Autodesk Inventor part; units mm, degrees
ref_plane "Work Plane2" through (-40.9959, 0.8639, 22.2359) normal (0, 0, 1) x (1, 0, 0)
ref_plane "YZ Plane" through (0, 0, 0) normal (1, 0, 0) x (0, 1, 0)
ref_plane "XZ Plane" through (0, 0, 0) normal (0, 1, 0) x (-1, 0, 0)
ref_plane "Work Plane1" through (0, 0, 10) normal (0, 0, 1) x (1, 0, 0)
sketch "Sketch1" plane through (0, 0, 10) normal (0, 0, 1) x (1, 0, 0)
  line L0 (-4.0299, -0.3538) -> (-2.2322, 1.4439) construction
  arc A0 (-1.4439, 2.2322) -> (-2.2322, 1.4439) centre (-0.9299, 0.9299) ccw construction
  line L1 (-1.4439, 2.2322) -> (0.3538, 4.0299) construction
  line L2 (-37.8299, 42.8299) -> (-37.8299, 37.8299) construction
  line L3 (-37.8299, 37.8299) -> (-42.9208, 37.8299) construction
  line L4 (-37.8299, 42.2137) -> (-37.8299, 45.8299) construction
  line L5 (-37.8299, 45.8299) -> (-4.0299, 45.8299) construction
  line L6 (-4.0299, 45.8299) -> (-4.0299, 42.2137) construction
  line L7 (-4.0299, 4.0299) -> (0.3538, 4.0299)
  circle A1 centre (-20.9299, 20.9299) radius 17.5
  line L8 (-20.9299, 58.9723) -> (17.1124, 20.9299) construction
  line L9 (17.1124, 20.9299) -> (-20.9299, -17.1124) construction
  line L10 (-20.9299, -17.1124) -> (-58.9723, 20.9299) construction
  line L11 (-58.9723, 20.9299) -> (-20.9299, 58.9723) construction
  line L12 (-20.9299, 58.9723) -> (-20.9299, -17.1124) construction
  line L13 (17.1124, 20.9299) -> (-58.9723, 20.9299) construction
  line L14 (-20.9299, 58.9723) -> (32.8701, 58.9723) construction
  line L15 (-43.4299, 43.4299) -> (1.5701, 43.4299) construction
  line L16 (1.5701, 43.4299) -> (1.5701, -1.5701) construction
  line L17 (1.5701, -1.5701) -> (-43.4299, -1.5701) construction
  line L18 (-43.4299, -1.5701) -> (-43.4299, 43.4299) construction
  line L19 (-43.4299, 43.4299) -> (1.5701, -1.5701) construction
  line L20 (1.5701, 43.4299) -> (-43.4299, -1.5701) construction
  line L21 (-43.4299, 5.3876) -> (-43.4299, 36.4723)
  line L22 (-43.4299, 36.4723) -> (-36.4723, 43.4299)
  line L23 (-36.4723, 43.4299) -> (-5.3876, 43.4299)
  line L24 (-5.3876, 43.4299) -> (1.5701, 36.4723)
  line L25 (1.5701, 36.4723) -> (1.5701, 5.3876)
  line L26 (1.5701, 5.3876) -> (-5.3876, -1.5701)
  line L27 (-5.3876, -1.5701) -> (-36.4723, -1.5701)
  line L28 (-36.4723, -1.5701) -> (-43.4299, 5.3876)
  line L29 (-4.0299, 42.2137) -> (-37.8299, 42.2137)
  line L30 (-4.0299, -0.3538) -> (-4.0299, 4.0299)
  point P0 (-37.8299, 4.0299)
  point P1 (-20.9299, 20.9299)
  dimension "d18" = 53.8
  dimension "d19" = 45
  dimension "d20" = 53.8
  dimension "d21" = 45
  dimension "d22" = 45
extrude "Extrusion1" add sketch "Sketch1" along normal blind 8
sketch "Sketch2" plane through (0, 0, 18) normal (0, 0, 1) x (1, 0, 0)
  circle A0 centre (-35.9299, 35.9299) radius 3.0099 construction
  circle A1 centre (-5.93, 35.9299) radius 3.0099 construction
  circle A2 centre (-5.93, 5.93) radius 3.0099 construction
  circle A3 centre (-35.9299, 5.93) radius 3.0099 construction
  circle A4 centre (-35.9299, 35.9299) radius 2.95
  circle A5 centre (-5.93, 35.9299) radius 2.95
  circle A6 centre (-5.93, 5.93) radius 2.95
  circle A7 centre (-35.9299, 5.93) radius 2.95
  point P0 (0, 0)
  dimension "d1" = 5.9
  dimension "d31" = 5.9
  dimension "d32" = 5.9
  dimension "d33" = 5.9
ref_plane "Work Plane2" through (-40.9959, 0.8639, 22.2359) normal (0, 0, 1) x (1, 0, 0)
extrude "Extrusion2" add sketch "Sketch2" along normal blind 8
sketch "Sketch3" plane through (0, 0, 10) normal (0, 0, -1) x (-1, 0, 0)
  line L0 (37.8299, -0.4701) -> (37.8299, 4.0299) construction
  line L1 (4.0299, 4.0299) -> (4.0299, -0.4701) construction
  line L2 (37.8299, -0.4701) -> (37.8299, 1.1886) construction
  line L3 (4.0299, -3.9701) -> (4.0299, -0.3538) construction
  line L4 (45.8299, 4.0299) -> (42.2137, 4.0299) construction
  line L5 (-0.3538, 4.0299) -> (-3.9701, 4.0299) construction
  line L6 (-3.9701, 37.8299) -> (-0.3538, 37.8299) construction
  line L7 (4.0299, 42.2137) -> (4.0299, 45.8299) construction
  line L8 (37.8299, 45.8299) -> (37.8299, 42.2137) construction
  line L9 (42.2137, 37.8299) -> (45.8299, 37.8299) construction
  line L10 (40.4657, 37.7299) -> (45.8299, 37.7299)
  line L11 (45.8299, 37.7299) -> (45.8299, 4.1299)
  line L12 (45.8299, 4.1299) -> (40.4657, 4.1299)
  line L13 (40.4657, 4.1299) -> (40.4657, 37.7299)
  line L14 (37.7299, 2.4952) -> (4.1299, 2.4952)
  line L15 (4.1299, 2.4952) -> (4.1299, -3.9701)
  line L16 (4.1299, -3.9701) -> (37.7299, -3.9701)
  line L17 (37.7299, -3.9701) -> (37.7299, 2.4952)
  line L18 (1.8946, 4.1299) -> (-3.9701, 4.1299)
  line L19 (-3.9701, 4.1299) -> (-3.9701, 37.7299)
  line L20 (-3.9701, 37.7299) -> (1.8946, 37.7299)
  line L21 (1.8946, 37.7299) -> (1.8946, 4.1299)
  line L22 (4.1299, 40.7326) -> (37.7299, 40.7326)
  line L23 (37.7299, 40.7326) -> (37.7299, 45.8299)
  line L24 (37.7299, 45.8299) -> (4.1299, 45.8299)
  line L25 (4.1299, 45.8299) -> (4.1299, 40.7326)
  point P0 (0, 0)
  dimension "d23" = 0.1
  dimension "d24" = 0.1
  dimension "d25" = 0.1
  dimension "d26" = 0.1
  dimension "d27" = 0.1
extrude "Extrusion3" add sketch "Sketch3" against normal up to surface (8 mm away)
sketch "Sketch4" plane through (0, 0, 18) normal (0, 0, 1) x (1, 0, 0)
  line L0 (3.9701, 4.1299) -> (0.3124, 4.1299)
  line L1 (3.9701, 37.7299) -> (3.9701, 4.1299)
  line L2 (0.3124, 37.7299) -> (3.9701, 37.7299)
  line L3 (0.3124, 37.7299) -> (-4.1299, 42.1723)
  line L4 (-4.1299, 45.8299) -> (-4.1299, 42.1723)
  line L5 (-37.7299, 45.8299) -> (-4.1299, 45.8299)
  line L6 (-37.7299, 42.1723) -> (-37.7299, 45.8299)
  line L7 (-37.7299, 42.1723) -> (-42.1723, 37.7299)
  line L8 (-45.8299, 37.7299) -> (-42.1723, 37.7299)
  line L9 (-45.8299, 4.1299) -> (-45.8299, 37.7299)
  line L10 (-42.1723, 4.1299) -> (-45.8299, 4.1299)
  line L11 (-42.1723, 4.1299) -> (-37.7299, -0.3124)
  line L12 (-37.7299, -3.9701) -> (-37.7299, -0.3124)
  line L13 (-4.1299, -3.9701) -> (-37.7299, -3.9701)
  line L14 (-4.1299, -0.3124) -> (-4.1299, -3.9701)
  line L15 (-4.1299, -0.3124) -> (0.3124, 4.1299)
  circle A0 centre (-20.9299, 20.9299) radius 17.5
  circle A1 centre (-35.9299, 5.93) radius 2.95
  circle A2 centre (-5.93, 35.9299) radius 2.95
  circle A3 centre (-35.9299, 35.9299) radius 2.95
  circle A4 centre (-5.93, 5.93) radius 2.95
  line L16 (-3.9799, 45.9799) -> (-3.9799, 42.2344)
  line L17 (-3.9799, 42.2344) -> (0.3745, 37.8799)
  line L18 (0.3745, 37.8799) -> (4.1201, 37.8799)
  line L19 (4.1201, 37.8799) -> (4.1201, 3.9799)
  line L20 (4.1201, 3.9799) -> (0.3745, 3.9799)
  line L21 (0.3745, 3.9799) -> (-3.9799, -0.3745)
  line L22 (-3.9799, -0.3745) -> (-3.9799, -4.1201)
  line L23 (-3.9799, -4.1201) -> (-37.8799, -4.1201)
  line L24 (-37.8799, -4.1201) -> (-37.8799, -0.3745)
  line L25 (-37.8799, -0.3745) -> (-42.2344, 3.9799)
  line L26 (-42.2344, 3.9799) -> (-45.9799, 3.9799)
  line L27 (-45.9799, 3.9799) -> (-45.9799, 37.8799)
  line L28 (-45.9799, 37.8799) -> (-42.2344, 37.8799)
  line L29 (-42.2344, 37.8799) -> (-37.8799, 42.2344)
  line L30 (-37.8799, 42.2344) -> (-37.8799, 45.9799)
  line L31 (-37.8799, 45.9799) -> (-3.9799, 45.9799)
  point P0 (0, 0)
  dimension "d34" = 0.15
extrude "Extrusion4" add sketch "Sketch4" against normal up to surface (8 mm away) contours L16 L17 L18 L19 L20 L21 L22 L23 L24 L25 L26 L27 L28 L29 L30 L31
ref_plane "Arbeitsebene3" through (-37.8799, 20.9299, 18) normal (0, -1, 0) x (1, 0, 0)
ref_plane "Arbeitsebene4" through (-20.9299, 3.9799, 18) normal (1, 0, 0) x (0, 0, -1)
equation "\"d31\" = d1"
equation "\"d32\" = d1"
equation "\"d33\" = d1"
properties part number "20_Cube_Insert_Thorlabs_Pins"
For this review, take the finished solid that the model builds, in its own axes (mm). A direction names the side the tool comes from. Round coordinates to 2 decimals unless told otherwise and drop trailing zeros. Write each loop counter-clockwise with the first axis right and the second up, starting at its lowest first coordinate (ties: lowest second). Pieces come first, ordered by that corner, then holes. Notation, with made-up numbers: (-29, 42.25) - (5, 42.25) arc R22 ccw to (5, 54.25) - close; hole circle Ø1 at (-7, 73.5). An arc over 180 degrees is marked (long way). Answer as a JSON object with one key per item and string values.
1. We need section A-A on x = -27. Give the boundary of the cut face in (y, z), then the cut area to 3 significant figures.
Response values:
{"outline": "(-4.12, 10) - (4.52, 10) - (4.52, 18) - (-4.12, 18) - close; (37.34, 10) - (45.98, 10) - (45.98, 18) - (37.34, 18) - close", "area": "138 mm2"}
2. Tool access review of faces 1 (the face through (-44, 37.88, 14)), 2 (the face through (2, 37.88, 14)), 3 (the face through (2, 3.98, 14)), 4 (the face through (-37.88, -2, 14)), 5 (the face through (-4.569, 38.547, 21.944)): name each direction out of +Z, -Z, +X, -X, +Y, -Y from which nothing blocks a thin tool from reaching the whole face with its end or side.
Response values:
{"face 1": "+Z, -Z, -X, +Y", "face 2": "+Z, -Z, +X, +Y", "face 3": "+Z, -Z, +X, -Y", "face 4": "+Z, -Z, -X, -Y", "face 5": "+Z"}
3. We need section C-C on z = 16.75. Give the boundary of the cut face in (x, y).
Response values:
{"outline": "(-45.98, 3.98) - (-42.23, 3.98) - (-37.88, -0.37) - (-37.88, -4.12) - (-3.98, -4.12) - (-3.98, -0.37) - (0.37, 3.98) - (4.12, 3.98) - (4.12, 37.88) - (0.37, 37.88) - (-3.98, 42.23) - (-3.98, 45.98) - (-37.88, 45.98) - (-37.88, 42.23) - (-42.23, 37.88) - (-45.98, 37.88) - close; hole circle Ø35 at (-20.93, 20.93)"}
4. Draft analysis for pull direction X (two halves, no side actions). For faces 6 (the face through (-38.271, 37.725, 21.944)), 7 (the face through (-3.116, 5.044, 21.944)), 8 (the face through (-44, 3.98, 14)), 9 (the face through (4.12, 21, 14)), state which applies: +X half, -X half, draft (parallel to the pull), parting line (faces both ways), or undercut.
Response values:
{"face 6": "undercut", "face 7": "undercut", "face 8": "draft", "face 9": "+X half"}
5. To check wall thickness, follow line 1 along Y through (x, z) = (-20.5, 12); line 2 along Z through (x, y) = (-5.5, 11.5); line 3 along Y through (x, z) = (-12.5, 13.5). State the ranges of each line that lie inside material, in increasing order.
Response values:
{"line 1": "y = -4.12 to 3.44, 38.42 to 45.98", "line 2": "z = 10 to 18", "line 3": "y = -4.12 to 5.59, 36.27 to 45.98"}
6. For pin 1 Ø4 at (y, z) = (43.5, 14) entering from +X; pin 2 Ø5 at (y, z) = (10.5, 22) entering from +X; pin 3 Ø3 at (x, z) = (-43, 15) entering from -Y, all flat-tipped, find the tip position at first contact; note any pin that passes through.
Response values:
{"pin 1": "stops at x = -3.25", "pin 2": "stops at x = -3.83", "pin 3": "stops at y = 3.25"}
7. We need section D-D on y = 34. Give the boundary of the cut face in (x, z).
Response values:
{"outline": "(-45.98, 10) - (-32.57, 10) - (-32.57, 18) - (-33.7, 18) - (-33.7, 26) - (-38.16, 26) - (-38.16, 18) - (-45.98, 18) - close; (-9.29, 10) - (4.12, 10) - (4.12, 18) - (-3.7, 18) - (-3.7, 26) - (-8.16, 26) - (-8.16, 18) - (-9.29, 18) - close"}
8. We need section B-B on y = 14.5. Give the boundary of the cut face in (x, z), then the cut area to 3 significant figures.
Response values:
{"outline": "(-45.98, 10) - (-37.21, 10) - (-37.21, 18) - (-45.98, 18) - close; (-4.65, 10) - (4.12, 10) - (4.12, 18) - (-4.65, 18) - close", "area": "140 mm2"}
